Here's how the part is built. I have some questions about the finished solid (model axes, mm). A direction names the side the tool comes from. Coordinates: 2 decimals unless noted, no trailing zeros. Loops run counter-clockwise (first coordinate to the right, second up) from the corner with the lowest first, then second, coordinate; pieces in that order, holes last. Notation, with made-up numbers: (18, 18) - (66, 18) arc R16 cw to (66, 44) - close; hole circle Ø3 at (-3, -27.5). An arc over 180 degrees is marked (long way). Use a Markdown table: item, result.
Autodesk Inventor part; units mm, degrees
ref_plane "YZ Plane" through (0, 0, 0) normal (1, 0, 0) x (0, 1, 0)
ref_plane "XZ Plane" through (0, 0, 0) normal (0, 1, 0) x (-1, 0, 0)
ref_plane "XY Plane" through (0, 0, 0) normal (0, 0, 1) x (1, 0, 0)
sketch "Sketch1" plane through (0, 0, 0) normal (0, 0, 1) x (1, 0, 0)
  line L0 (0, 0) -> (0, -25)
  line L1 (0, 0) -> (2.75, 0)
  line L2 (2.75, 0) -> (4, -1.25)
  line L3 (4, -1.25) -> (4, -25)
  line L4 (4, -25) -> (0, -25)
  dimension "d0" = 8
  dimension "d1" = 5.5
  dimension "d2" = 45
  dimension "d14" = 25
revolve "Вращение1" add sketch "Sketch1" angle 360 about axis through (0, 0, 0) along (0, -1, 0)
thread "Резьба1"
sketch "Sketch2" plane through (0, 0, 0) normal (0, 0, 1) x (1, 0, 0)
  line L0 (-0.6, 0) -> (0.6, 0)
  line L1 (0.6, 0) -> (0.6, -2.5)
  line L2 (0.6, -2.5) -> (-0.6, -2.5)
  line L3 (-0.6, -2.5) -> (-0.6, 0)
  line L4 (0, 0) -> (0, -2.5)
  dimension "d9" = 1.2
  dimension "d10" = 2.5
extrude "Выдавливание1" cut sketch "Sketch2" along normal through all both and the other way through all
chamfer "Фаска1" distance 1.25 angle 45 1 edges at (-4, -25, 0)
equation "\"d9\" = n"
equation "\"d10\" = t"
equation "\"d19\" = -0.5 * dp + 0.5 * d_"
equation "\"d0\" = d_"
equation "\"d1\" = df_"
equation "\"d2\" = an"
equation "\"d14\" = l_"
equation "\"df_\" = 5.5"
equation "\"t\" = 2.5"
equation "\"n\" = 1.2"
equation "\"d_\" = 8"
equation "\"dp\" = 5.5"
equation "\"l_\" = 25"
equation "\"an\" = 45deg"
properties part number "Винт M8-6gx25 ГОСТ 1477-93" material "Сталь, мягкая"
Q1. I want a section at C-C, the plane y = -4. Write out the boundary of the cut face in (x, z).
Check values:
| item | result |
|---|---|
| outline | circle Ø8 at (0, 0) |
Q2. Will these pins go through, and if not, where does the flat tip stop? P1, Ø1.5, axis at x = -1.5, y = -18, coming from the -Z side; P2, Ø3, axis at y = -5, z = 3, coming from the +X side; P3, Ø2, axis at x = -2.5, y = -8.5, coming from the -Z side.
Check values:
| item | result |
|---|---|
| P1 | z = -3.93 |
| P2 | x = 3.71 |
| P3 | z = -3.71 |
Q3. Which directions (+Z, -Z, +X, -X, +Y, -Y) give clear straight access to the entire face, cutting with the end or side of a thin tool? Please do faces 5 (the face through (0, -25, 0)), 6 (the face through (0, -2.5, 0)).
Check values:
| item | result |
|---|---|
| face 5 | +Z, -Z, +X, -X, -Y |
| face 6 | +Z, -Z, +Y |
Q4. If we mould it in two halves opening along X, with no side actions, what happens to faces 1 (the face through (-2.97, -0.22, 0.06)), 2 (the face through (1, 0, 0)), 3 (the face through (-0.6, -1, 0)), 4 (the face through (0.6, -1, 0))? For each: pulls with the +X half, pulls with the -X half, needs draft (parallel to the pull), parting line crosses it, or undercut.
Check values:
| item | result |
|---|---|
| face 1 | pulls with the -X half |
| face 2 | needs draft |
| face 3 | undercut |
| face 4 | undercut |
Q5. Please list where these lines run through material, in increasing order: L1, parallel to X at y = -2, z = 0.25; L2, parallel to Y at x = -0.5, z = 1.5; L3, parallel to Y at x = 3, z = -1.5. Write a range as from..to.
Check values:
| item | result |
|---|---|
| L1 | -3.99..-0.6, 0.6..3.99 |
| L2 | -25..-2.5 |
| L3 | -24.4..-0.6 |
Q6. I want a section at B-B, the plane x = 0. Write out the boundary of the cut face in (y, z).
Check values:
| item | result |
|---|---|
| outline | (-25, -2.75) - (-23.75, -4) - (-2.5, -4) - (-2.5, 4) - (-23.75, 4) - (-25, 2.75) - close |
Q7. I want a section at A-A, the plane z = 0. Write out the boundary of the cut face in (x, y), then the cut area to 3 significant figures.
Check values:
| item | result |
|---|---|
| outline | (-4, -23.75) - (-2.75, -25) - (2.75, -25) - (4, -23.75) - (4, -1.25) - (2.75, 0) - (0.6, 0) - (0.6, -2.5) - (-0.6, -2.5) - (-0.6, 0) - (-2.75, 0) - (-4, -1.25) - close |
| area | 194 mm^2 |
